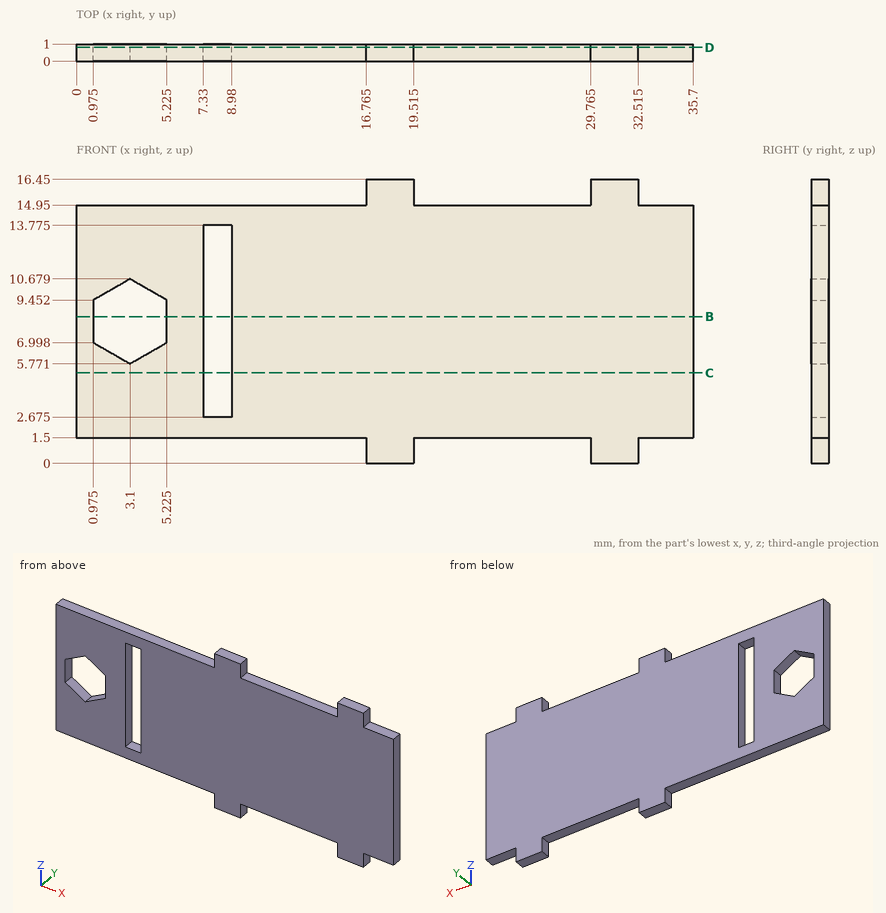
Part print with two shaded views. Sizes in mm from the minimum x, y, z corner. Round coordinates to 2 decimals unless told otherwise and drop trailing zeros. Order: outer loops, then holes, each group sorted by start corner. A loop starts at its lowest first (then second) coordinate and runs counter-clockwise, first axis right, second up. Notation, with made-up numbers: (13, 68.5) - (40, 68.5) arc R7 cw to (40, 78.5) - close; hole circle Ø11 at (87.5, 12). An arc over 180 degrees is marked (long way). Return JSON: item names as keys, results as strings.
(1) Wall check: probe 1 along X at (y, z) = (0.65, 8.5) (1 decimal); probe 2 along X at (y, z) = (0.15, 11.75); probe 3 along X at (y, z) = (0.55, 9.5). Give the ranges that are in metal, low to high. Write a range as from..to.
Answer key:
{"probe 1": "x = 0..1, 5.2..7.3, 9..35.7", "probe 2": "x = 0..7.33, 8.98..35.7", "probe 3": "x = 0..1.06, 5.14..7.33, 8.98..35.7"}
(2) Pin check, flat tips, straight feed: pin 1 Ø0.5 at (x, y) = (4.5, 0.5) entering from -Z; pin 2 Ø1.5 at (x, z) = (30.5, 8.5) entering from -Y. Stop position of each tip, or through.
Answer key:
{"pin 1": "stops at z = 1.5", "pin 2": "stops at y = 0"}
(3) Cut at B-B (z = 8.5). Give the cut face in (x, y) (1 decimal).
Answer key:
{"outline": "(0, 0) - (1, 0) - (1, 1) - (0, 1) - close; (5.2, 0) - (7.3, 0) - (7.3, 1) - (5.2, 1) - close; (9, 0) - (35.7, 0) - (35.7, 1) - (9, 1) - close"}
(4) Cut at C-C (z = 5.25). Give the cut face in (x, y).
Answer key:
{"outline": "(0, 0) - (7.33, 0) - (7.33, 1) - (0, 1) - close; (8.98, 0) - (35.7, 0) - (35.7, 1) - (8.98, 1) - close"}
(5) Cut at D-D (y = 0.8). State how many separate pieces and enclosed holes the cut face has, then the cut area to 3 significant figures.
Answer key:
{"separate pieces": "1", "enclosed holes": "2", "area": "463 mm^2"}
